from build123d import *

# Parameters (mm, degrees)
BOSS_EXTRUDE1_DEPTH   = 69.85
F_4_CLEARANCE_HOLE1_D = 3.2639
F_4_CLEARANCE_HOLE2_D = 3.2639


with BuildPart() as part:
    # Sketch1 → Boss-Extrude1 (new body)
    with BuildSketch(Plane.XY):
        Polygon((0, 0), (0, 19.05), (1.5875, 19.05), (1.5875, 1.5875), (19.05, 1.5875), (19.05, 0), align=None)
    extrude(amount=BOSS_EXTRUDE1_DEPTH)

    # #4 Clearance Hole1 (through all)
    with Locations(Plane(origin=(1.5875, 0, 0), x_dir=(0, 0, -1), z_dir=(1, 0, 0))):
        with Locations((-63.5, 9.525)):
            Hole(F_4_CLEARANCE_HOLE1_D / 2)

    # #4 Clearance Hole2 (through all)
    with Locations(Plane(origin=(0, 1.5875, 0), x_dir=(1, 0, 0), z_dir=(0, 1, 0))):
        with Locations((9.525, -12.7), (9.807915651, -31.75)):
            Hole(F_4_CLEARANCE_HOLE2_D / 2)


solid = part.part
The model under review builds one solid part; all positions refer to its coordinate system, in mm. A direction names the side the tool comes from. Round coordinates to 2 decimals unless told otherwise and drop trailing zeros. Write each loop counter-clockwise with the first axis right and the second up, starting at its lowest first coordinate (ties: lowest second). Pieces come first, ordered by that corner, then holes. Notation, with made-up numbers: (70.25, -36.75) - (114.25, -36.75) arc R7 cw to (114.25, -32.75) - close; hole circle Ø5 at (12.25, 39). An arc over 180 degrees is marked (long way). One line per item, written item: value. Start each with the question number.
1. Clearance check with flat-ended pins moving along their axes: P1, Ø4, axis at x = 9.525, z = 12.7, coming from the -Y side; P2, Ø8.5, axis at x = 9.5, z = 39, coming from the +Y side; P3, Ø2, axis at y = 9.525, z = 63.5, coming from the -X side (3 decimals). State where each tip first meets the part, or that it passes through.
2. The part is to be moulded in two halves that separate along X. For faces 1 (the face through (19.05, 1, 34)), 2 (the face through (10.162, 0.783, 33.343)), 3 (the face through (1, 19.05, 34)), say which applies: released by +X, released by -X, zero draft, split by the parting line, or undercut.
3. Machinability: for faces 4 (the face through (1.588, 10, 34)), 5 (the face through (5, 1, 69.85)), which of the approach directions +Z, -Z, +X, -X, +Y, -Y give a long, thin tool a straight path to every point of the face, cutting with its end or side? Answer none if there is none.
4. Consider section C-C on x = 4. Write out the cut boundary in (y, z), and give its area (3 significant figures).
5. Consider section A-A on z = 12. Write out the cut boundary in (x, y), and give its area (3 significant figures).
6. To check wall thickness, follow L1, parallel to X at y = 1.2, z = 12.7; L2, parallel to X at y = 1.75, z = 41.5. State the ranges of each line that lie inside material, in increasing order. Write a range as from..to.
7. Consider section B-B on z = 26. Write out the cut boundary in (x, y).
Checks:
1. P1: stops at y = 0
1. P2: stops at y = 1.59
1. P3: passes through
2. face 1: released by +X
2. face 2: undercut
2. face 3: zero draft
3. face 4: +Z, -Z, +X, +Y
3. face 5: +Z, +X, -X, +Y, -Y
4. outline: (0, 0) - (1.59, 0) - (1.59, 69.85) - (0, 69.85) - close
4. area: 111 mm^2
5. outline: (0, 0) - (8.05, 0) - (8.05, 1.59) - (1.59, 1.59) - (1.59, 19.05) - (0, 19.05) - close; (11, 0) - (19.05, 0) - (19.05, 1.59) - (11, 1.59) - close
5. area: 53.3 mm^2
6. L1: x = 0..7.89, 11.16..19.05
6. L2: x = 0..1.59
7. outline: (0, 0) - (19.05, 0) - (19.05, 1.59) - (1.59, 1.59) - (1.59, 19.05) - (0, 19.05) - close
